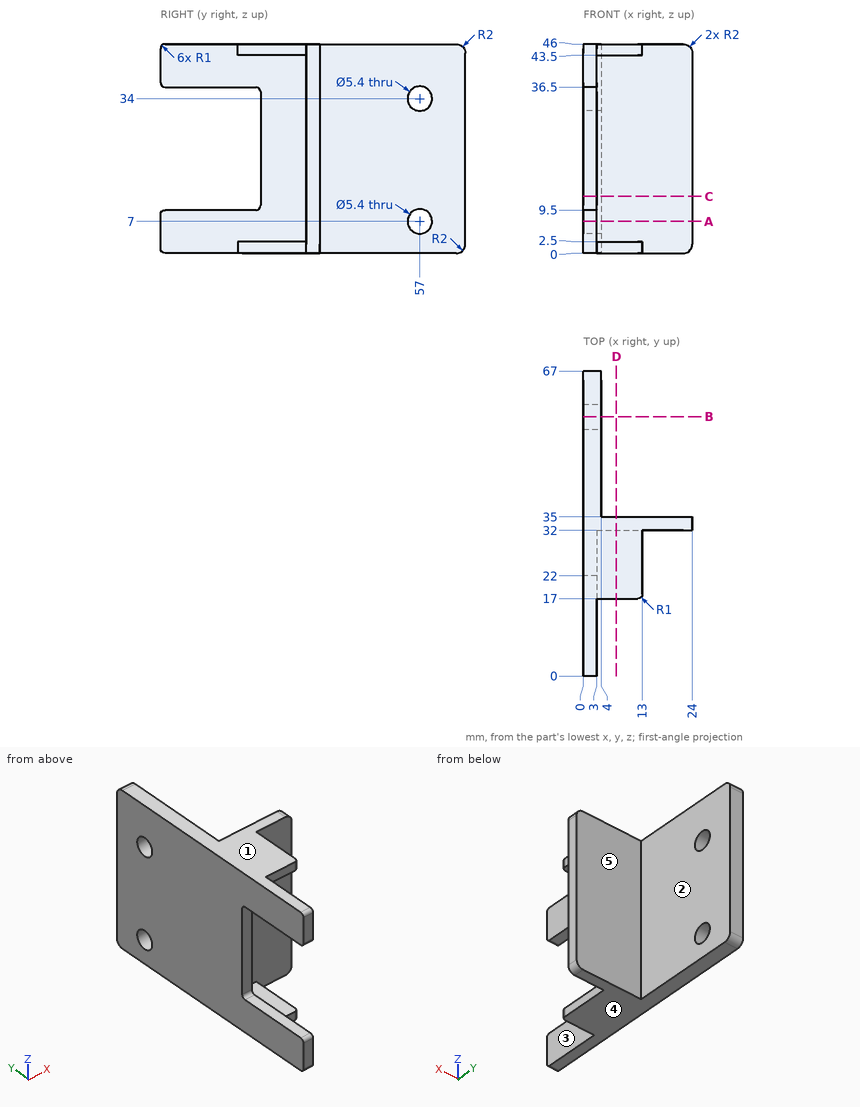
Input: dimensioned drawing with shaded views. Units: mm. Origin: part minimum x, y, z. A direction names the side the tool comes from. Coordinates: 2 decimals unless noted, no trailing zeros. Order: outer loops, then holes, each group sorted by start corner. A loop starts at its lowest first (then second) coordinate and runs counter-clockwise, first axis right, second up. Notation, with made-up numbers: (41.5, 77) -> (56.5, 77) arc R28 cw to (56.5, 111) -> close; hole circle Ø9 at (-30, 6.5). An arc over 180 degrees is marked (long way). Answer in a Markdown table with one row per item.
Item 1: Section C-C on z = 12.5. Output: boundary loops of the cut face in (x, y).
Return value:
| item | result |
|---|---|
| outline | (0, 22) -> (3, 22) -> (3, 32) -> (24, 32) -> (24, 35) -> (4, 35) -> (4, 67) -> (0, 67) -> close |
Item 2: Section D-D on x = 7.25. Output: boundary loops of the cut face in (y, z).
Return value:
| item | result |
|---|---|
| outline | (17, 0) -> (35, 0) -> (35, 46) -> (17, 46) -> (17, 43.5) -> (32, 43.5) -> (32, 2.5) -> (17, 2.5) -> close |
Item 3: Section B-B on y = 57. Output: boundary loops of the cut face in (x, z).
Return value:
| item | result |
|---|---|
| outline | (0, 0) -> (4, 0) -> (4, 4.3) -> (0, 4.3) -> close; (0, 9.7) -> (4, 9.7) -> (4, 31.3) -> (0, 31.3) -> close; (0, 36.7) -> (4, 36.7) -> (4, 46) -> (0, 46) -> close |
Item 4: Ray query, L1, parallel to Z at x = 3.75, y = 59; L2, parallel to Y at x = 2.25, z = 34; L3, parallel to Y at x = 6.75, z = 26.5. Return the intervals inside material, ascending.
Return value:
| item | result |
|---|---|
| L1 | z = 0 to 5.19, 8.81 to 32.19, 35.81 to 46 |
| L2 | y = 22 to 54.3, 59.7 to 67 |
| L3 | y = 32 to 35 |
Item 5: Draft query along Z for the marked faces 3, 4 and 5. Return one class per face: released by +Z, released by -Z, zero draft, split by the parting line, or undercut.
Return value:
| item | result |
|---|---|
| face 3 | undercut |
| face 4 | released by -Z |
| face 5 | zero draft |
Item 6: Access query for the marked faces 1 and 2. Directions: +Z, -Z, +X, -X, +Y, -Y. A direction counts if a zero-diameter tool reaches every point of the face in a straight line with its end or side. Return the directions, or none.
Return value:
| item | result |
|---|---|
| face 1 | +Z, +X, -X, +Y, -Y |
| face 2 | +Z, -Z, +X, +Y |
Item 7: Contact query for flat-ended pins moving along their axis: P1, Ø10, axis at x = 10.5, z = 11, coming from the +Y side; P2, Ø2, axis at y = 26, z = 45, coming from the +X side; P3, Ø16, axis at y = 53.5, z = 26, coming from the +X side; P4, Ø4.5, axis at y = 57, z = 7, coming from the +X side. Output: stop coordinate, or through.
Return value:
| item | result |
|---|---|
| P1 | stops at y = 35 |
| P2 | stops at x = 13 |
| P3 | stops at x = 4 |
| P4 | passes through |
Item 8: Section A-A on z = 7. Output: boundary loops of the cut face in (x, y).
Return value:
| item | result |
|---|---|
| outline | (0, 0) -> (3, 0) -> (3, 32) -> (24, 32) -> (24, 35) -> (4, 35) -> (4, 54.3) -> (0, 54.3) -> close; (0, 59.7) -> (4, 59.7) -> (4, 67) -> (0, 67) -> close |
